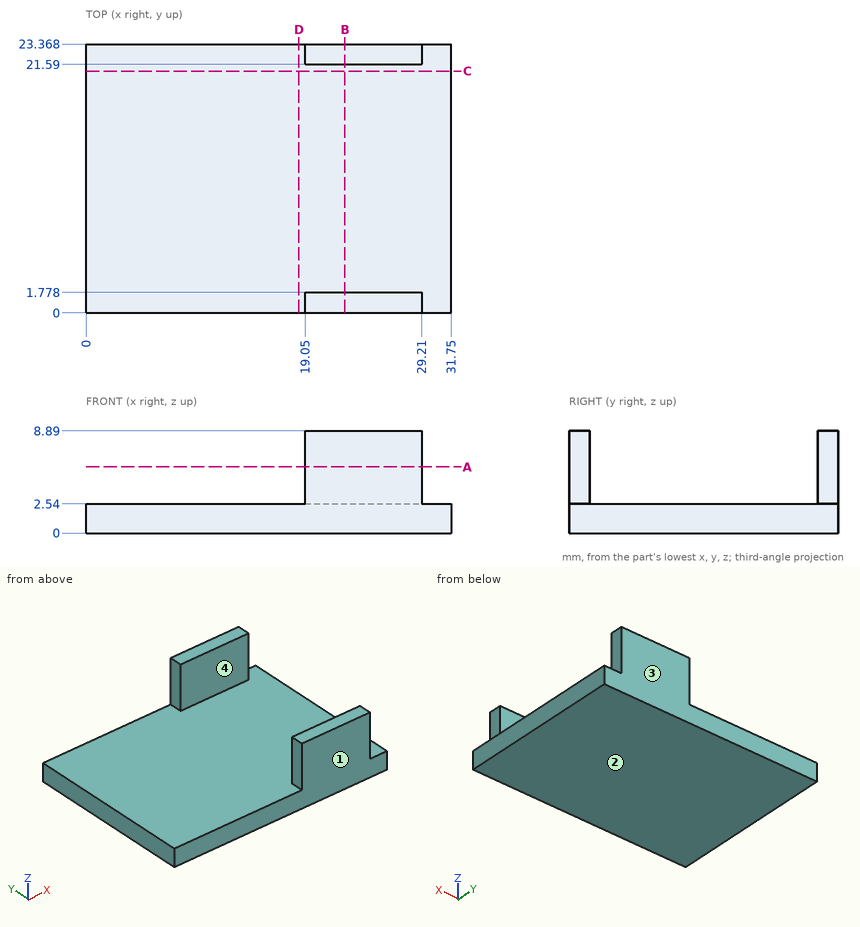
Verification items for this drawing (mm, ordinates from the low corner). Round coordinates to 2 decimals unless told otherwise and drop trailing zeros. Write each loop counter-clockwise with the first axis right and the second up, starting at its lowest first coordinate (ties: lowest second). Pieces come first, ordered by that corner, then holes. Notation, with made-up numbers: (57.5, -22.75) - (96.5, -22.75) arc R9 ccw to (96.5, -9.75) - close; hole circle Ø2 at (-25, 48). An arc over 180 degrees is marked (long way). One line per item, written item: value.
1. Cross-section at B-B on x = 22.5. Record the boundary of the cut face in (y, z).
The answers:
outline: (0, 0) - (23.37, 0) - (23.37, 8.89) - (21.59, 8.89) - (21.59, 2.54) - (1.78, 2.54) - (1.78, 8.89) - (0, 8.89) - close
2. Scan lines: L1, parallel to Y at x = 24.5, z = 7.5; L2, parallel to Z at x = 10, y = 5.25; L3, parallel to X at y = 22.75, z = 4. Record each from-to range of solid material in increasing order.
The answers:
L1: y = 0 to 1.78, 21.59 to 23.37
L2: z = 0 to 2.54
L3: x = 19.05 to 29.21
3. Cross-section at C-C on y = 21. Record the boundary of the cut face in (x, z), and give its area (3 significant figures).
The answers:
outline: (0, 0) - (31.75, 0) - (31.75, 2.54) - (0, 2.54) - close
area: 80.6 mm^2
4. Cross-section at D-D on x = 18.5. Record the boundary of the cut face in (y, z), and give its area (3 significant figures).
The answers:
outline: (0, 0) - (23.37, 0) - (23.37, 2.54) - (0, 2.54) - close
area: 59.4 mm^2
5. Cross-section at A-A on z = 5.75. Record the boundary of the cut face in (x, y), and give its area (3 significant figures).
The answers:
outline: (19.05, 0) - (29.21, 0) - (29.21, 1.78) - (19.05, 1.78) - close; (19.05, 21.59) - (29.21, 21.59) - (29.21, 23.37) - (19.05, 23.37) - close
area: 36.1 mm^2
6. Mould release check, pull along Y, two halves, no side actions. Record for the marked faces 1, 2, 3 and 4: released by +Y, released by -Y, zero draft, split by the parting line, or undercut.
The answers:
face 1: released by -Y
face 2: zero draft
face 3: released by +Y
face 4: undercut
7. Depth check by flat-ended pin: pin 1 Ø2 at (y, z) = (22.5, 7.5) entering from +X; pin 2 Ø1.5 at (y, z) = (20, 4) entering from +X; pin 3 Ø2 at (y, z) = (22.5, 7) entering from -X; pin 4 Ø8 at (x, y) = (4.5, 16.5) entering from +Z. Enter the tip coordinate at first touch or a pass-through.
The answers:
pin 1: stops at x = 29.21
pin 2: passes through
pin 3: stops at x = 19.05
pin 4: stops at z = 2.54
